```python
from build123d import *

# Parameters (mm, degrees)
BOX_W             = 10
BOX_H             = 10
BOX_DEPTH         = 10
SKETCH_W          = 4.4
SKETCH_H          = 4.4
PAD_DEPTH         = 4
PAD_FACE1_W       = 10
PAD_FACE1_H       = 10
POCKET_DEPTH      = 2.5
POCKET_FACE3_W    = 10
POCKET_FACE3_H    = 10
POCKET001_DEPTH   = 2.5
POCKET001_FACE6_W = 5
POCKET001_FACE6_H = 10
PAD001_DEPTH      = 10
SKETCH001_W       = 4.4
SKETCH001_H       = 4.4
PAD002_DEPTH      = 4
PAD002_FACE3_W    = 10
PAD002_FACE3_H    = 10
PAD003_DEPTH      = 10
PAD003_FACE16_W   = 10
PAD003_FACE16_H   = 10
PAD004_DEPTH      = 10
PAD004_FACE19_W   = 10
PAD004_FACE19_H   = 10
POCKET002_DEPTH   = 10
POCKET002_FACE9_W = 10
POCKET002_FACE9_H = 10
POCKET003_DEPTH   = 10


with BuildPart() as part:
    # Box → Box (new body)
    with BuildSketch(Plane.XY):
        with Locations((5, 5)):
            Rectangle(BOX_W, BOX_H)
    extrude(amount=BOX_DEPTH)

    # Sketch (on Face6 of BaseFeature) → Pad (new body)
    with BuildSketch(Plane.XY.offset(10)):
        with Locations((5, 5)):
            Rectangle(SKETCH_W, SKETCH_H)
    extrude(amount=PAD_DEPTH)

    # Pad Face1 → Pocket (cut)
    with BuildSketch(Plane(origin=(0, 5, 5), x_dir=(0, 1, 0), z_dir=(-1, 0, 0))):
        Rectangle(PAD_FACE1_W, PAD_FACE1_H)
    extrude(amount=-POCKET_DEPTH, mode=Mode.SUBTRACT)

    # Pocket Face3 → Pocket001 (cut)
    with BuildSketch(Plane(origin=(10, 5, 5), x_dir=(0, -1, 0), z_dir=(1, 0, 0))):
        Rectangle(POCKET_FACE3_W, POCKET_FACE3_H)
    extrude(amount=-POCKET001_DEPTH, mode=Mode.SUBTRACT)

    # Pocket001 Face6 → Pad001 (add)
    with BuildSketch(Plane(origin=(5, 10, 5), x_dir=(1, 0, 0), z_dir=(0, 1, 0))):
        Rectangle(POCKET001_FACE6_W, POCKET001_FACE6_H)
    extrude(amount=PAD001_DEPTH)

    # Sketch001 (on Face8 of Pad001) → Pad002 (join)
    with BuildSketch(Plane.XY.offset(10)):
        with Locations((5, 15)):
            Rectangle(SKETCH001_W, SKETCH001_H)
    extrude(amount=PAD002_DEPTH)

    # Pad002 Face3 → Pad003 (add)
    with BuildSketch(Plane(origin=(7.5, 5, 5), x_dir=(0, -1, 0), z_dir=(1, 0, 0))):
        Rectangle(PAD002_FACE3_W, PAD002_FACE3_H)
    extrude(amount=PAD003_DEPTH)

    # Pad003 Face16 → Pad004 (add)
    with BuildSketch(Plane(origin=(7.5, 15, 5), x_dir=(0, -1, 0), z_dir=(1, 0, 0))):
        Rectangle(PAD003_FACE16_W, PAD003_FACE16_H)
    extrude(amount=PAD004_DEPTH)

    # Pad004 Face19 → Pocket002 (cut)
    with BuildSketch(Plane(origin=(17.5, 15, 5), x_dir=(0, -1, 0), z_dir=(1, 0, 0))):
        Rectangle(PAD004_FACE19_W, PAD004_FACE19_H)
    extrude(amount=-POCKET002_DEPTH, mode=Mode.SUBTRACT)

    # Pocket002 Face9 → Pocket003 (cut)
    with BuildSketch(Plane(origin=(17.5, 5, 5), x_dir=(0, -1, 0), z_dir=(1, 0, 0))):
        Rectangle(POCKET002_FACE9_W, POCKET002_FACE9_H)
    extrude(amount=-POCKET003_DEPTH, mode=Mode.SUBTRACT)


solid = part.part
```
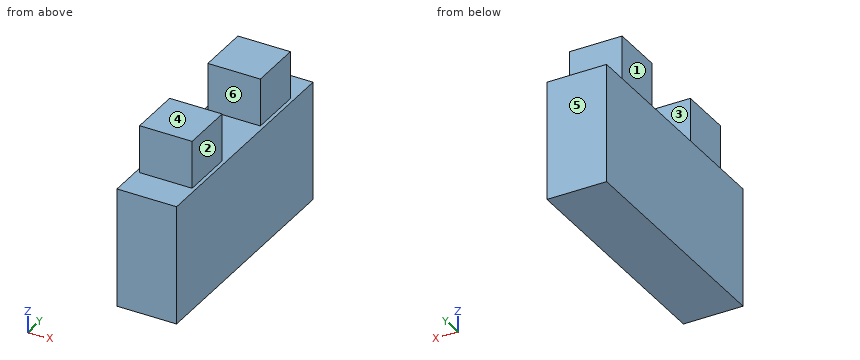
Source: CAD feature listing. Evaluate the final solid. Frame: model axes, mm. Face numbers are marked on the shaded views. A direction names the side the tool comes from. Round coordinates to 2 decimals unless told otherwise and drop trailing zeros. Loops run counter-clockwise (first coordinate to the right, second up) from the corner with the lowest first, then second, coordinate; pieces in that order, holes last. Notation, with made-up numbers: M -7.5,30 L 12.5,30 A34 cw 12.5,61 Z; hole C 72.25,1 d7. An arc over 180 degrees is marked long. Use a Markdown table: item, result. Add a question column.
1. Cut plane C-C, the plane x = 4. Output: boundary loops of the cut face in (y, z).
2. Cut plane A-A, the plane z = 12.5. Output: boundary loops of the cut face in (x, y).
3. Contact query for flat-ended pins moving along their axis: pin 1 (4.5 mm diameter, centred on y = 15, z = 12.5, fed in from -X); pin 2 (1.5 mm diameter, centred on x = 6.5, z = 12, fed in from -Y); pin 3 (3 mm diameter, centred on y = 6, z = 12, fed in from +X). Output: stop coordinate, or through.
4. Ray query, line 1 along Y through (x, z) = (4.5, 12.5); line 2 along Z through (x, y) = (3.2, 9); line 3 along X through (y, z) = (5.75, 10.25). Return the intervals inside material, ascending. Write a range as [from, to].
5. Cut plane B-B, the plane y = 14.75. Output: boundary loops of the cut face in (x, z).
6. Pull-direction query (Y, two-part tool) for the marked faces 4, 5 and 6; classes: +Y half, -Y half, draft (parallel to the pull), parting line (faces both ways), or undercut.
7. Set-up query: the marked faces 1, 2 and 3. Return all of +Z, -Z, +X, -X, +Y, -Y with unobstructed straight access to the full face (end or side cutting, diameter ignored); none if empty.
8. Cut plane D-D, the plane y = 12.5. Output: boundary loops of the cut face in (x, z), and give its area (3 significant figures).
Solution:
| question | item | result |
|---|---|---|
| 1 | outline | M 0,0 L 20,0 L 20,10 L 17.2,10 L 17.2,14 L 12.8,14 L 12.8,10 L 7.2,10 L 7.2,14 L 2.8,14 L 2.8,10 L 0,10 Z |
| 2 | outline | M 2.8,2.8 L 7.2,2.8 L 7.2,7.2 L 2.8,7.2 Z; M 2.8,12.8 L 7.2,12.8 L 7.2,17.2 L 2.8,17.2 Z |
| 3 | pin 1 | stops at x = 2.8 |
| 3 | pin 2 | stops at y = 2.8 |
| 3 | pin 3 | stops at x = 7.2 |
| 4 | line 1 | y = [2.8, 7.2], [12.8, 17.2] |
| 4 | line 2 | z = [0, 10] |
| 4 | line 3 | x = [2.8, 7.2] |
| 5 | outline | M 2.5,0 L 7.5,0 L 7.5,10 L 7.2,10 L 7.2,14 L 2.8,14 L 2.8,10 L 2.5,10 Z |
| 6 | face 4 | draft |
| 6 | face 5 | +Y half |
| 6 | face 6 | undercut |
| 7 | face 1 | +Z, -X, +Y, -Y |
| 7 | face 2 | +Z, +X, +Y, -Y |
| 7 | face 3 | +Z, +X, -X |
| 8 | outline | M 2.5,0 L 7.5,0 L 7.5,10 L 2.5,10 Z |
| 8 | area | 50.0 mm2 |
